from build123d import *

# Parameters (mm, degrees)
F0_R     = 3.96875
F1_DEPTH = 19.05
F3_DEPTH = 19.05


with BuildPart() as f1:
    # F0 (on Front) → F1 (new body)
    with BuildSketch(Plane.XZ):
        with BuildLine():
            Line((-9.525, 0), (-9.525, -9.525))
            Line((-9.525, -9.525), (0, -9.525))
            ThreePointArc((0, -9.525), (-6.7351920908, -6.7351920908), (-9.525, 0))
        make_face()
        with BuildLine():
            ThreePointArc((9.525, 0), (6.7351920908, -6.7351920908), (0, -9.525))
            Line((0, -9.525), (9.525, -9.525))
            Line((9.525, -9.525), (9.525, 0))
        make_face()
        with BuildLine():
            ThreePointArc((-9.525, 0), (-6.7351920908, -6.7351920908), (0, -9.525))
            ThreePointArc((0, -9.525), (6.7351920908, -6.7351920908), (9.525, 0))
            ThreePointArc((9.525, 0), (6.7351920908, 6.7351920908), (0, 9.525))
            ThreePointArc((0, 9.525), (-6.7351920908, 6.7351920908), (-9.525, 0))
        make_face()
        Circle(F0_R, mode=Mode.SUBTRACT)
        with BuildLine():
            Line((-9.525, 9.525), (-9.525, 0))
            ThreePointArc((-9.525, 0), (-6.7351920908, 6.7351920908), (0, 9.525))
            Line((0, 9.525), (-9.525, 9.525))
        make_face()
        with BuildLine():
            ThreePointArc((0, 9.525), (6.7351920908, 6.7351920908), (9.525, 0))
            Line((9.525, 0), (9.525, 9.525))
            Line((9.525, 9.525), (0, 9.525))
        make_face()
    extrude(amount=F1_DEPTH)

    # F2 (on face) → F3 (cut)
    with BuildSketch(Plane.YZ.offset(9.525)):
        Polygon((-7.9375, -9.525), (-9.525, -7.9375), (-11.1125, -9.525), align=None)
    extrude(amount=-F3_DEPTH, mode=Mode.SUBTRACT)

    # F5 (on mid) → F6 (revolve, cut)
    with BuildSketch(Plane.YZ):
        Polygon((-19.05, 20.5410033949), (-19.05, 9.525), (-16.0982707865, 20.5410033949), align=None)
        Polygon((-2.9517292135, 20.5410033949), (0, 9.525), (0, 20.5410033949), align=None)
    revolve(axis=Axis((0, 0, 0), (0, 1, 0)), mode=Mode.SUBTRACT)


solid = f1.part
Design review of the part built by this model. Coordinates are the model's own, in mm. A direction names the side the tool comes from. Coordinates: 2 decimals unless noted, no trailing zeros. Order: outer loops, then holes, each group sorted by start corner. A loop starts at its lowest first (then second) coordinate and runs counter-clockwise, first axis right, second up. Notation, with made-up numbers: (-22.75, -7) -> (4.25, -7) arc R27 ccw to (4.25, 31) -> close; hole circle Ø9 at (65.25, -6.5). An arc over 180 degrees is marked (long way). Use one line per item in the form item = value. Start each with the question number.
(1) For probe 1 along Z at (x, y) = (0, -3.75) (3 decimals); probe 2 along X at (y, z) = (-2.5, 2.5) (3 decimals); probe 3 along Z at (x, y) = (1, -0.75) (3 decimals), list the stretches that pass through material, from the lowest coordinate up.
(2) The part is to be moulded in two halves that separate along X. For faces 3 (the cylindrical face through (-0.86, -9.392, -3.874)), 4 (the conical face through (-7.4, -18.8, 7.4)), 5 (the flat face through (0, -15, -9.525)), say which applies: +X half, -X half, draft (parallel to the pull), parting line (faces both ways), or undercut.
(3) Add section A-A on y = -6.25. State the section outline as (x, z) points (1 decimal), plus the area to 3 significant figures.
(4) For faces 1 (the conical face through (-7.4, -18.8, -7.4)), 2 (the flat face through (0.13, -8.72, -8.74)), list the 3-axis set-ups (+Z, -Z, +X, -X, +Y, -Y) from which the entire face can be reached by the end or side of a thin tool; tool diameter is ignored.
(5) Add section B-B on y = -10. State the section outline as (x, z) points (1 decimal), plus the area to 3 significant figures.
Answer block:
q1.probe_1 = -9.525 to -3.969, 3.969 to 9.525
q1.probe_2 = -9.525 to -3.082, 3.082 to 9.525
q1.probe_3 = -9.525 to -3.841, 3.841 to 9.525
q2.face_3 = undercut
q2.face_4 = -X half
q2.face_5 = draft
q3.outline = (-9.5, -9.5) -> (9.5, -9.5) -> (9.5, 9.5) -> (-9.5, 9.5) -> close; hole circle Ø7.9 at (0, 0)
q3.area = 313 mm²
q4.face_1 = -Z, -X, -Y
q4.face_2 = -Z, +X, -X
q5.outline = (-9.5, -8.4) -> (9.5, -8.4) -> (9.5, 9.5) -> (-9.5, 9.5) -> close; hole circle Ø7.9 at (0, 0)
q5.area = 292 mm²
